Input: part model. Units: mm. Frame: model coordinates. Face numbers are marked on the shaded views. A direction names the side the tool comes from. Round coordinates to 2 decimals unless told otherwise and drop trailing zeros. Loops run counter-clockwise (first coordinate to the right, second up) from the corner with the lowest first, then second, coordinate; pieces in that order, holes last. Notation, with made-up numbers: (0, 57.5) -> (31, 57.5) arc R11 cw to (31, 72.5) -> close; hole circle Ø11 at (78.5, 10). An arc over 180 degrees is marked (long way). Answer in a Markdown table with one row per item. Add a question column.
Q1. Section B-B, the plane y = 3.25. Output: boundary loops of the cut face in (x, z).
Q2. Reachability of the marked faces 4 and 5 from +Z, -Z, +X, -X, +Y, -Y: full face, straight path, thin tool, end or side. Return the list, or none.
Q3. Mould query, pull axis X, two halves, no side actions, for the marked faces 1, 2 and 3. Classes: pulls with the +X half, pulls with the -X half, needs draft (parallel to the pull), parting line crosses it, or undercut.
Q4. Section A-A, the plane x = 0. Output: boundary loops of the cut face in (y, z), and give its area (3 significant figures).
Q5. Ray query, L1, parallel to Y at x = 3, z = 1.5; L2, parallel to X at y = 6, z = 0; L3, parallel to Y at x = -1, z = -0.25. Return the intervals inside material, ascending. Write a range as from..to.
Q6. Pin query (flat end, axial travel): pin 1 (2 mm diameter, centred on x = -0.5, y = 2, fed in from -Z); pin 2 (2 mm diameter, centred on x = 0, y = 11.5, fed in from -Z); pin 3 (1.5 mm diameter, centred on y = 8, z = -2.5, fed in from -X). Return the tip coordinate at first contact, or that it passes through.
```python
from build123d import *

# Parameters (mm, degrees)
SKETCH1_R           = 4
BOSS_EXTRUDE1_DEPTH = 1.2
SKETCH2_R           = 2
BOSS_EXTRUDE2_DEPTH = 14
FILLET2_R           = 0.3
CUT_EXTRUDE1_DEPTH  = 0.6


with BuildPart() as part:
    # Sketch1 → Boss-Extrude1 (new body)
    with BuildSketch(Plane(origin=(0, 0, 0), x_dir=(1, 0, 0), z_dir=(0, 1, 0))):
        with Locations(Location((0, 0, 0), (0, 0, 270))):
            Circle(SKETCH1_R)
    extrude(amount=BOSS_EXTRUDE1_DEPTH)

    # Sketch2 → Boss-Extrude2 (add)
    with BuildSketch(Plane(origin=(0, 1.2, 0), x_dir=(1, 0, 0), z_dir=(0, 1, 0))):
        with Locations(Location((0, 0, 0), (0, 0, 270))):
            Circle(SKETCH2_R)
    extrude(amount=BOSS_EXTRUDE2_DEPTH)

    # Fillet2
    fillet2_edges = [part.edges().sort_by_distance(p)[0] for p in [
        (0, 0, -4),
        (0, 1.2, -4),
    ]]
    fillet(fillet2_edges, radius=FILLET2_R)

    # Sketch3 → Cut-Extrude1 (cut)
    with BuildSketch(Plane.XZ):
        Polygon((1.732050808, 0), (0.866025404, 1.5), (-0.866025404, 1.5), (-1.732050808, 0), (-0.866025404, -1.5), (0.866025404, -1.5), align=None)
    extrude(amount=-CUT_EXTRUDE1_DEPTH, mode=Mode.SUBTRACT)


solid = part.part
```
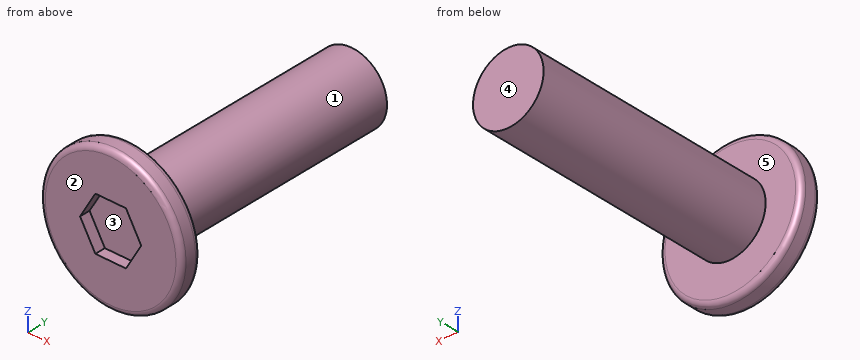
Answer block:
| question | item | result |
|---|---|---|
| 1 | outline | circle Ø4 at (0, 0) |
| 2 | face 4 | +Z, -Z, +X, -X, +Y |
| 2 | face 5 | +Y |
| 3 | face 1 | parting line crosses it |
| 3 | face 2 | needs draft |
| 3 | face 3 | undercut |
| 4 | outline | (0, -3.7) arc R0.3 ccw to (0.3, -4) -> (0.9, -4) arc R0.3 ccw to (1.2, -3.7) -> (1.2, -2) -> (15.2, -2) -> (15.2, 2) -> (1.2, 2) -> (1.2, 3.7) arc R0.3 ccw to (0.9, 4) -> (0.3, 4) arc R0.3 ccw to (0, 3.7) -> (0, 1.5) -> (0.6, 1.5) -> (0.6, -1.5) -> (0, -1.5) -> close |
| 4 | area | 63.7 mm^2 |
| 5 | L1 | 0..1.2 |
| 5 | L2 | -2..2 |
| 5 | L3 | 0.6..15.2 |
| 6 | pin 1 | z = -3.96 |
| 6 | pin 2 | z = -2 |
| 6 | pin 3 | x = -0.97 |
